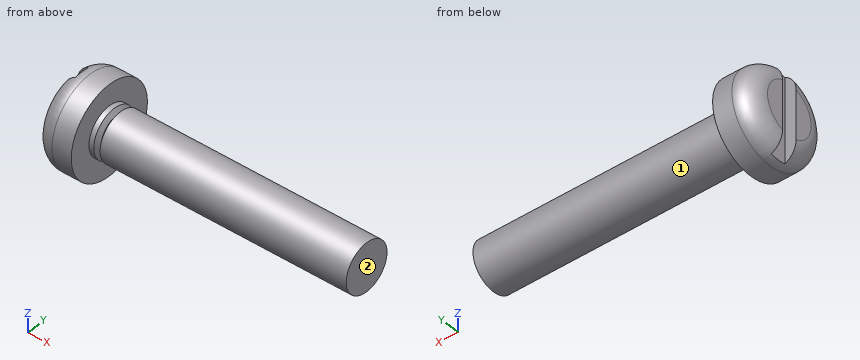
from build123d import *

# Parameters (mm, degrees)
SKETCH2_W  = 5.6
SKETCH2_H  = 1
SLOT_DEPTH = 0.7


with BuildPart() as part:
    # BodySke → Base-Revolve (revolve)
    with BuildSketch(Plane.XY, mode=Mode.PRIVATE) as base_revolve_sk:
        with BuildLine():
            Line((2.4, 1.5), (2.4, 2.8))
            Line((2.4, 2.8), (1.2, 2.8))
            ThreePointArc((1.2, 2.8), (0.351471863, 2.448528137), (0, 1.6))
            Line((0, 1.6), (0, 0))
            Line((0, 0), (18.4, 0))
            Line((18.4, 0), (18.4, 1.5))
            Line((18.4, 1.5), (2.4, 1.5))
        make_face()
    revolve(base_revolve_sk.sketch.rotate(Axis((-25.4, 0, 0), (1, 0, 0)), 90), axis=Axis((-25.4, 0, 0), (1, 0, 0)))

    # Sketch2 → Slot (cut)
    with BuildSketch(Plane(origin=(0, 0, 0), x_dir=(0, 0, -1), z_dir=(1, 0, 0))):
        Rectangle(SKETCH2_W, SKETCH2_H)
    extrude(amount=SLOT_DEPTH, mode=Mode.SUBTRACT)

    # ThdSchSke → ThreadSchematic (revolve, cut)
    with BuildSketch(Plane.XY):
        Polygon((2.9, -1.2195), (2.703591786, -1.5), (2.703591786, -1.875), (3.096408214, -1.875), (3.096408214, -1.5), align=None)
    revolve(axis=Axis((-3.175, 0, 0), (1, 0, 0)), mode=Mode.SUBTRACT)


solid = part.part
Model file for the job. Use its own axes, mm. Face numbers are marked on the shaded views. A direction names the side the tool comes from. Coordinates: 2 decimals unless noted, no trailing zeros. Write each loop counter-clockwise with the first axis right and the second up, starting at its lowest first coordinate (ties: lowest second). Pieces come first, ordered by that corner, then holes. Notation, with made-up numbers: (50.5, 31) -> (86.5, 31) arc R20 ccw to (86.5, 54) -> close; hole circle Ø9 at (8.5, 29.25). An arc over 180 degrees is marked (long way). One line per item, written item: value. Start each with the question number.
1) Flat gauge pins, fed straight in: pin 1 Ø0.8 at (y, z) = (0, 0.5) entering from -X; pin 2 Ø1.5 at (x, z) = (5.5, -1) entering from +Y; pin 3 Ø1 at (x, y) = (15.5, 0) entering from +Z. Where does each tip first touch, or does it go through?
2) Which spindle directions (+Z, -Z, +X, -X, +Y, -Y) get a long thin tool onto all of the face, cutting with end or side? Do the marked faces 1 and 2. Say none if no direction does.
3) Slice it at C-C on z = 0. Write the cut outline in (x, y).
4) Slice it at B-B on x = 3.75. Write the cut outline in (y, z).
5) Probe probe 1 along Y at (x, z) = (5.25, -0.1); probe 2 along X at (y, z) = (0.9, 1.45); probe 3 along Z at (x, y) = (1.75, 2.3). List the from-to ranges inside material, lowest first.
6) Slice it at A-A on y = 0. Write the cut outline in (x, z), then the cut area to 3 significant figures.
Answers follow:
1. pin 1: x = 0.7
1. pin 2: y = 1.48
1. pin 3: z = 1.5
2. face 1: +X
2. face 2: +Z, -Z, +X, +Y, -Y
3. outline: (0, -1.6) arc R1.2 ccw to (1.2, -2.8) -> (2.4, -2.8) -> (2.4, -1.5) -> (2.7, -1.5) -> (2.9, -1.22) -> (3.1, -1.5) -> (18.4, -1.5) -> (18.4, 1.5) -> (3.1, 1.5) -> (2.9, 1.22) -> (2.7, 1.5) -> (2.4, 1.5) -> (2.4, 2.8) -> (1.2, 2.8) arc R1.2 ccw to (0, 1.6) -> (0, 0.5) -> (0.7, 0.5) -> (0.7, -0.5) -> (0, -0.5) -> close
4. outline: circle Ø3 at (0, 0)
5. probe 1: -1.5 to 1.5
5. probe 2: 0 to 2.4
5. probe 3: -1.6 to 1.6
6. outline: (0.7, -2.69) arc R1.2 ccw to (1.2, -2.8) -> (2.4, -2.8) -> (2.4, -1.5) -> (2.7, -1.5) -> (2.9, -1.22) -> (3.1, -1.5) -> (18.4, -1.5) -> (18.4, 1.5) -> (3.1, 1.5) -> (2.9, 1.22) -> (2.7, 1.5) -> (2.4, 1.5) -> (2.4, 2.8) -> (1.2, 2.8) arc R1.2 ccw to (0.7, 2.69) -> close
6. area: 57.4 mm2
